Work out the finished part from the listing and answer in its coordinate system (mm). A direction names the side the tool comes from. Coordinates: 2 decimals unless noted, no trailing zeros. Order: outer loops, then holes, each group sorted by start corner. A loop starts at its lowest first (then second) coordinate and runs counter-clockwise, first axis right, second up. Notation, with made-up numbers: M 56,87 L 76,87 A23 ccw 76,120 Z; hole C 67,7 d1. An arc over 180 degrees is marked long. Use a Markdown table: item, result.
from build123d import *

# Parameters (mm, degrees)
SKETCH1_W           = 38
SKETCH1_H           = 20
BOSS_EXTRUDE1_DEPTH = 31
SKETCH2_W           = 35
SKETCH2_H           = 17
CUT_EXTRUDE1_DEPTH  = 28
SKETCH3_W           = 6
SKETCH3_H           = 17
BOSS_EXTRUDE2_DEPTH = 17.5
SKETCH4_W           = 42
SKETCH4_H           = 24
SKETCH4_W_2         = 38
SKETCH4_H_2         = 20
EXTRUDE_THIN2_DEPTH = 1.4
SKETCH5_R           = 1
CUT_EXTRUDE2_DEPTH  = 3
SKETCH6_R           = 1
CUT_EXTRUDE3_DEPTH  = 3
SKETCH7_W           = 8
SKETCH7_H           = 3
CUT_EXTRUDE4_DEPTH  = 10
SKETCH8_W           = 18
SKETCH8_H           = 9
CUT_EXTRUDE5_DEPTH  = 2
SKETCH9_R           = 3.725
SKETCH9_R_2         = 0.7
CUT_EXTRUDE6_DEPTH  = 4
FILLET1_R           = 4


with BuildPart() as part:
    # Sketch1 → Boss-Extrude1 (new body)
    with BuildSketch(Plane(origin=(0, 0, 0), x_dir=(1, 0, 0), z_dir=(0, 1, 0))):
        with Locations((8.6, -4.057142857)):
            Rectangle(SKETCH1_W, SKETCH1_H)
    extrude(amount=BOSS_EXTRUDE1_DEPTH)

    # Sketch2 → Cut-Extrude1 (cut)
    with BuildSketch(Plane(origin=(0, 31, 0), x_dir=(1, 0, 0), z_dir=(0, 1, 0))):
        with Locations((8.5, -3.957142857)):
            Rectangle(SKETCH2_W, SKETCH2_H)
    extrude(amount=-CUT_EXTRUDE1_DEPTH, mode=Mode.SUBTRACT)

    # Sketch3 → Boss-Extrude2 (add)
    with BuildSketch(Plane(origin=(0, 3, 0), x_dir=(1, 0, 0), z_dir=(0, 1, 0))):
        with Locations((-6, -3.957142857)):
            Rectangle(SKETCH3_W, SKETCH3_H)
        with Locations((23, -3.957142857)):
            Rectangle(SKETCH3_W, SKETCH3_H)
    extrude(amount=BOSS_EXTRUDE2_DEPTH)

    # Sketch4 → Extrude-Thin2 (add)
    with BuildSketch(Plane(origin=(0, 31, 0), x_dir=(1, 0, 0), z_dir=(0, 1, 0))):
        with Locations((8.6, -4.057142857)):
            Rectangle(SKETCH4_W, SKETCH4_H)
        with Locations((8.6, -4.057142857)):
            Rectangle(SKETCH4_W_2, SKETCH4_H_2, mode=Mode.SUBTRACT)
    extrude(amount=-EXTRUDE_THIN2_DEPTH)

    # Sketch5 → Cut-Extrude2 (cut)
    with BuildSketch(Plane(origin=(0, 20.5, 0), x_dir=(1, 0, 0), z_dir=(0, 1, 0))):
        with Locations(Location((-5.5, -3.892148731, 0), (0, 0, 270))):
            Circle(SKETCH5_R)
    extrude(amount=-CUT_EXTRUDE2_DEPTH, mode=Mode.SUBTRACT)

    # Sketch6 → Cut-Extrude3 (cut)
    with BuildSketch(Plane(origin=(0, 20.5, 0), x_dir=(1, 0, 0), z_dir=(0, 1, 0))):
        with Locations(Location((22.953148274, -4.115727136, 0), (0, 0, 270))):
            Circle(SKETCH6_R)
    extrude(amount=-CUT_EXTRUDE3_DEPTH, mode=Mode.SUBTRACT)

    # Sketch7 → Cut-Extrude4 (cut)
    with BuildSketch(Plane(origin=(-3, 0, 0), x_dir=(0, 0, -1), z_dir=(1, 0, 0))):
        with Locations((-5.039117413, 5.541369126)):
            Rectangle(SKETCH7_W, SKETCH7_H)
    extrude(amount=-CUT_EXTRUDE4_DEPTH, mode=Mode.SUBTRACT)

    # Sketch8 → Cut-Extrude5 (cut)
    with BuildSketch(Plane(origin=(0, 3, 0), x_dir=(1, 0, 0), z_dir=(0, 1, 0))):
        with Locations((8.91134377, -3.084544202)):
            Rectangle(SKETCH8_W, SKETCH8_H)
    extrude(amount=-CUT_EXTRUDE5_DEPTH, mode=Mode.SUBTRACT)

    # Sketch9 → Cut-Extrude6 (cut)
    with BuildSketch(Plane(origin=(0, 1, 0), x_dir=(1, 0, 0), z_dir=(0, 1, 0))):
        with Locations(Location((8.68865623, -3.170580553, 0), (0, 0, 270))):
            Circle(SKETCH9_R)
        with Locations(Location((1.96365623, -3.170580553, 0), (0, 0, 270))):
            Circle(SKETCH9_R_2)
        with Locations(Location((15.41365623, -3.170580553, 0), (0, 0, 270))):
            Circle(SKETCH9_R_2)
    extrude(amount=-CUT_EXTRUDE6_DEPTH, mode=Mode.SUBTRACT)

    # Fillet1
    fillet1_edges = [part.edges().sort_by_distance(p)[0] for p in [
        (-0.08865623, 2, 7.584544202),
        (-0.08865623, 2, -1.415455798),
        (17.91134377, 2, -1.415455798),
        (17.91134377, 2, 7.584544202),
    ]]
    fillet(fillet1_edges, radius=FILLET1_R)


solid = part.part
1. Section B-B on y = 26.5 is taken. Determine the outline of the cut face in (x, z), then the cut area to 3 significant figures.
Answers below:
| item | result |
|---|---|
| outline | M -10.4,-5.94 L 27.6,-5.94 L 27.6,14.06 L -10.4,14.06 Z; hole M -9,-4.54 L 26,-4.54 L 26,12.46 L -9,12.46 Z |
| area | 165 mm² |
2. Flat-ended cylindrical pins translate along their axes: P1, Ø1.5, axis at x = -8, y = 5.5, coming from the +Z side; P2, Ø0.5, axis at y = 2, z = 3, coming from the +X side; P3, Ø1, axis at x = -7.5, y = 18.5, coming from the -Z side; P4, Ø1.3, axis at x = 15.41, z = 3.17, coming from the -Y side. Find the tip coordinate at first contact, or state that the pin passes through.
Answers below:
| item | result |
|---|---|
| P1 | z = 14.06 |
| P2 | x = 27.6 |
| P3 | z = -5.94 |
| P4 | through |
3. Section D-D on z = 13 is taken. Determine the outline of the cut face in (x, y), then the cut area to 3 significant figures.
Answers below:
| item | result |
|---|---|
| outline | M -12.4,29.6 L -10.4,29.6 L -10.4,0 L 27.6,0 L 27.6,29.6 L 29.6,29.6 L 29.6,31 L -12.4,31 Z |
| area | 1,180 mm² |
4. For faces 1 (the face through (16.108, 0.507, 3.079)), 2 (the face through (-10.4, 15, 4)), 3 (the face through (-3, 12, 4)), determine the directions among +Z, -Z, +X, -X, +Y, -Y from which every point of the face is accessible in a straight line to the end or side of a thin tool.
Answers below:
| item | result |
|---|---|
| face 1 | +Y, -Y |
| face 2 | +Z, -Z, -X, -Y |
| face 3 | +Y |
5. Section C-C on x = -5.5 is taken. Determine the outline of the cut face in (y, z).
Answers below:
| item | result |
|---|---|
| outline | M 0,-5.94 L 29.6,-5.94 L 29.6,-7.94 L 31,-7.94 L 31,-4.54 L 20.5,-4.54 L 20.5,2.89 L 17.5,2.89 L 17.5,4.89 L 20.5,4.89 L 20.5,12.46 L 31,12.46 L 31,16.06 L 29.6,16.06 L 29.6,14.06 L 0,14.06 Z; hole M 4.04,1.04 L 7.04,1.04 L 7.04,9.04 L 4.04,9.04 Z |
6. For a pull along X with two mould halves and no side action, classify faces 4 (the face through (7, 29.6, 15)), 5 (the face through (16.771, 1.986, -0.213)), 6 (the face through (-12.4, 30, 4)), 7 (the face through (-9, 26, 4)) as +X half, -X half, draft (parallel to the pull), parting line (faces both ways), or undercut.
Answers below:
| item | result |
|---|---|
| face 4 | draft |
| face 5 | undercut |
| face 6 | -X half |
| face 7 | undercut |
7. Find the intervals of material crossed by probe 1 along X at (y, z) = (8, 9.25); probe 2 along X at (y, z) = (23, 5); probe 3 along Z at (x, y) = (24.5, 22), in increasing order.
Answers below:
| item | result |
|---|---|
| probe 1 | -10.4 to -3, 20 to 27.6 |
| probe 2 | -10.4 to -9, 26 to 27.6 |
| probe 3 | -5.94 to -4.54, 12.46 to 14.06 |
8. Section A-A on z = 8.5 is taken. Determine the outline of the cut face in (x, y).
Answers below:
| item | result |
|---|---|
| outline | M -12.4,29.6 L -10.4,29.6 L -10.4,7.04 L -3,7.04 L -3,20.5 L -9,20.5 L -9,31 L -12.4,31 Z; M -10.4,0 L 27.6,0 L 27.6,29.6 L 29.6,29.6 L 29.6,31 L 26,31 L 26,20.5 L 20,20.5 L 20,3 L -3,3 L -3,4.04 L -10.4,4.04 Z |
